For this review, take the finished solid that the model builds, in its own axes (mm). Coordinates: 2 decimals unless noted, no trailing zeros. Loops run counter-clockwise (first coordinate to the right, second up) from the corner with the lowest first, then second, coordinate; pieces in that order, holes last. Notation, with made-up numbers: M 70,21.5 L 113,21.5 A7 cw 113,30.5 Z; hole C 4,88 d9. An arc over 180 degrees is marked long. Write item = value, one per line.
from build123d import *

# Parameters (mm, degrees)
BOSS_EXTRUDE1_DEPTH = 1
SKETCH2_R           = 0.5
CUT_EXTRUDE1_DEPTH  = 1


with BuildPart() as part:
    # Sketch1 → Boss-Extrude1 (new body)
    with BuildSketch(Plane.XY):
        with BuildLine():
            Line((0.566665575, 10.621911003), (4.836785257, 10.041508622))
            ThreePointArc((4.836785257, 10.041508622), (6.355848418, 8.75345876), (5.826769046, 6.833380545))
            ThreePointArc((5.826769046, 6.833380545), (3.832723198, 4.833381254), (2.062195705, 2.633052095))
            ThreePointArc((2.062195705, 2.633052095), (1.400201905, 1.530760177), (0.930843559, 0.333686241))
            ThreePointArc((0.930843559, 0.333686241), (0.837560316, 0.276531253), (0.770614998, 0.363057438))
            ThreePointArc((0.770614998, 0.363057438), (0.491345948, 3.315426366), (-0.739361897, 6.013542688))
            ThreePointArc((-0.739361897, 6.013542688), (-1.001481879, 6.56165987), (-1.091488982, 7.162524291))
            Line((-1.091488982, 7.162524291), (-1.091488982, 10.448413118))
            ThreePointArc((-1.091488982, 10.448413118), (-0.97227959, 10.710781676), (-0.696246031, 10.793568229))
            Line((-0.696246031, 10.793568229), (0.566665575, 10.621911003))
        make_face()
    extrude(amount=BOSS_EXTRUDE1_DEPTH)

    # Sketch2 → Cut-Extrude1 (cut)
    with BuildSketch(Plane.XY.offset(1)):
        with Locations((4.58754209, 8.207783975)):
            Circle(SKETCH2_R)
    extrude(amount=-CUT_EXTRUDE1_DEPTH, mode=Mode.SUBTRACT)


solid = part.part
Q1. Draft analysis for pull direction Y (two halves, no side actions). For faces 1 (the face through (-0.999, 6.554, 0.493)), 2 (the face through (0.5, 3.28, 0.49)), 3 (the face through (-1.091, 8.8, 0.5)), state which applies: +Y half, -Y half, draft (parallel to the pull), parting line (faces both ways), or undercut.
Solved:
face_1 = -Y half
face_2 = undercut
face_3 = draft
Q2. Add section A-A (x = 4.5). Write out the cut boundary in (y, z), and give its area (3 significant figures).
Solved:
outline = M 5.55,0 L 7.72,0 L 7.72,1 L 5.55,1 Z; M 8.7,0 L 10.09,0 L 10.09,1 L 8.7,1 Z
area = 3.55 mm²
Q3. Add section B-B (z = 0.45). Write out the cut boundary in (x, y).
Solved:
outline = M -1.09,7.16 A2.05 ccw -0.74,6.01 A8.93 cw 0.77,0.36 A0.08 ccw 0.93,0.33 A7.7 cw 2.06,2.63 A26.57 cw 5.83,6.83 A1.85 ccw 4.84,10.04 L -0.7,10.79 A0.35 ccw -1.09,10.45 Z; hole C 4.59,8.21 d1
Q4. Add section C-C (y = 8.5). Write out the cut boundary in (x, z).
Solved:
outline = M -1.09,0 L 4.18,0 L 4.18,1 L -1.09,1 Z; M 4.99,0 L 6.41,0 L 6.41,1 L 4.99,1 Z
Q5. For line 1 along X through (y, z) = (8.25, 0.35); line 2 along X through (y, z) = (8.5, 0.8); line 3 along X through (y, z) = (7, 0.8), list the stretches that pass through material, from the lowest coordinate up.
Solved:
line_1 = -1.09 to 4.09, 5.09 to 6.44
line_2 = -1.09 to 4.18, 4.99 to 6.41
line_3 = -1.09 to 5.99
Q6. Add section D-D (x = 0.25). Write out the cut boundary in (y, z), and give its area (3 significant figures).
Solved:
outline = M 4.08,0 L 10.66,0 L 10.66,1 L 4.08,1 Z
area = 6.59 mm²
